Part print with two shaded views. Sizes in mm from the minimum x, y, z corner. Coordinates: 2 decimals unless noted, no trailing zeros. Write each loop counter-clockwise with the first axis right and the second up, starting at its lowest first coordinate (ties: lowest second). Pieces come first, ordered by that corner, then holes.
Q1. Drill centre lines: probe 1 along Y at (x, z) = (27.5, 7.5); probe 2 along Y at (x, z) = (15, 6); probe 3 along Y at (x, z) = (57, 11). Where is each one in solid material? Low to high.
Q2. Band-saw the part on C-C, the plane z = 7.5. Write the cut outline in (x, y).
Q3. Band-saw the part on B-B, the plane y = 40.66. Write the cut outline in (x, z).
Q4. Band-saw the part on D-D, the plane y = 7. Write the cut outline in (x, z).
Q5. Band-saw the part on A-A, the plane x = 15. Write the cut outline in (y, z).
Q6. Pull direction Y, two halves, no side cores. Call the marked faces 1, 2 and 3: released by +Y, released by -Y, zero draft, split by the parting line, or undercut.
Q7. Pin check, flat tips, straight feed: P1, Ø12, axis at x = 34.5, y = 40.5, coming from the -Z side; P2, Ø20, axis at x = 15, y = 40.66, coming from the +Z side. Stop position of each tip, or through.
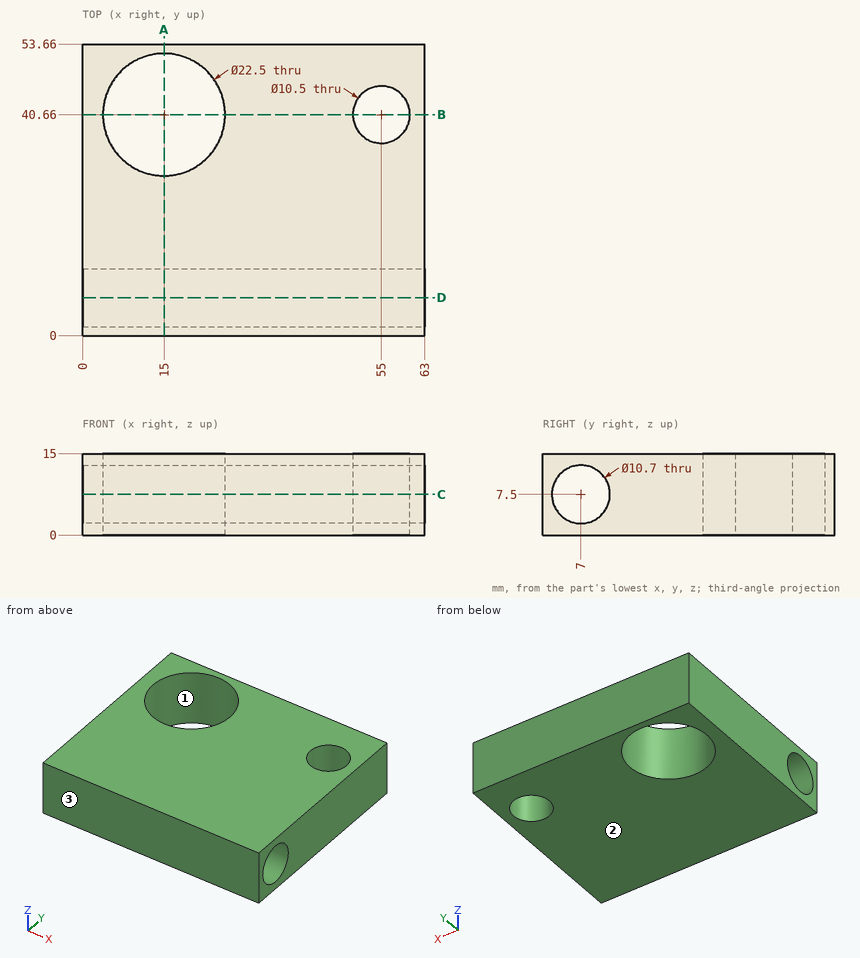
Answer sheet:
1. probe 1: y = 0 to 1.65, 12.35 to 53.66
1. probe 2: y = 0 to 1.86, 12.14 to 29.41, 51.91 to 53.66
1. probe 3: y = 0 to 2.95, 11.05 to 35.81, 45.51 to 53.66
2. outline: (0, 0) - (63, 0) - (63, 1.65) - (0, 1.65) - close; (0, 12.35) - (63, 12.35) - (63, 53.66) - (0, 53.66) - close; hole circle Ø22.5 at (15, 40.66); hole circle Ø10.5 at (55, 40.66)
3. outline: (0, 0) - (3.75, 0) - (3.75, 15) - (0, 15) - close; (26.25, 0) - (49.75, 0) - (49.75, 15) - (26.25, 15) - close; (60.25, 0) - (63, 0) - (63, 15) - (60.25, 15) - close
4. outline: (0, 0) - (63, 0) - (63, 2.15) - (0, 2.15) - close; (0, 12.85) - (63, 12.85) - (63, 15) - (0, 15) - close
5. outline: (0, 0) - (29.41, 0) - (29.41, 15) - (0, 15) - close; (51.91, 0) - (53.66, 0) - (53.66, 15) - (51.91, 15) - close; hole circle Ø10.7 at (7, 7.5)
6. face 1: undercut
6. face 2: zero draft
6. face 3: released by -Y
7. P1: stops at z = 0
7. P2: passes through
